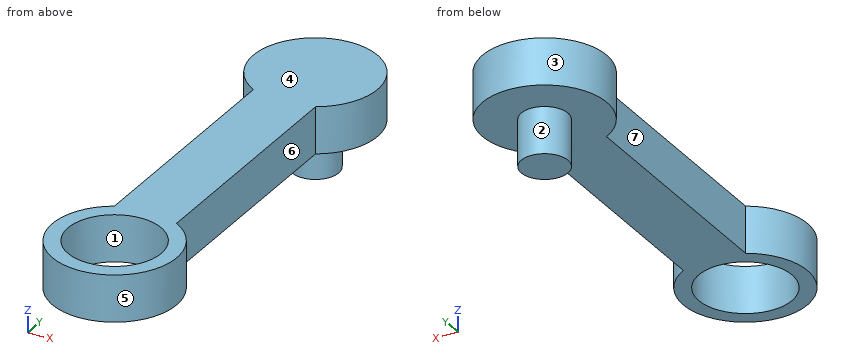
Autodesk Inventor part; units mm, degrees
ref_plane "YZ Plane" through (0, 0, 0) normal (1, 0, 0) x (0, 1, 0)
ref_plane "XZ Plane" through (0, 0, 0) normal (0, 1, 0) x (-1, 0, 0)
ref_plane "XY Plane" through (0, 0, 0) normal (0, 0, 1) x (1, 0, 0)
sketch "Sketch1" plane through (0, 0, 0) normal (0, 0, 1) x (1, 0, 0)
  arc A0 (-4, -15.5718) -> (4, -15.5718) centre (0, -22.5) ccw
  arc A1 (4, 15.5718) -> (-4, 15.5718) centre (0, 22.5) ccw
  line L0 (-4, 15.5718) -> (-4, -15.5718)
  line L1 (4, 15.5718) -> (4, -15.5718)
  circle A2 centre (0, 22.5) radius 3
  circle A3 centre (0, -22.5) radius 6
  point P0 (0, 0)
  dimension "d0" = 45
  dimension "d1" = 22.5
  dimension "d2" = 8
  dimension "d3" = 4
  dimension "d6" = 8
  dimension "d7" = 8
  dimension "d8" = 12
  dimension "d9" = 6
extrude "Extrusion1" add sketch "Sketch1" against normal blind 6
extrude "Extrusion2" add sketch "Sketch1" against normal blind 12 contours A2
properties part number "204"
Geometry: final body of the model. Coordinates: model frame, mm. Face numbers are marked on the shaded views. A direction names the side the tool comes from. Round coordinates to 2 decimals unless told otherwise and drop trailing zeros. Write each loop counter-clockwise with the first axis right and the second up, starting at its lowest first coordinate (ties: lowest second). Pieces come first, ordered by that corner, then holes. Notation, with made-up numbers: M 86.5,-3.5 L 131.5,-3.5 A26 ccw 131.5,33.5 Z; hole C 21.25,79.5 d4. An arc over 180 degrees is marked long. Answer in a Markdown table with one row per item. Add a question column.
(1) Cut plane B-B, the plane x = 0. Return the cut outline in (y, z), then the cut area to 3 significant figures.
(2) Cut plane C-C, the plane y = 22.5. Return the cut outline in (x, z).
(3) Draft query along Y for the marked faces 1, 2, 3 and 4. Return one class per face: pulls with the +Y half, pulls with the -Y half, needs draft (parallel to the pull), parting line crosses it, or undercut.
(4) Reachability of the marked faces 5, 6 and 7 from +Z, -Z, +X, -X, +Y, -Y: full face, straight path, thin tool, end or side. Return the list, or none.
(5) Ray query, L1, parallel to Y at x = 0, z = -2.55; L2, parallel to Z at x = -6, y = 18; L3, parallel to Y at x = 3.75, z = -1.25. Return the intervals inside material, ascending.
(6) Cut plane D-D, the plane z = -3. Return the cut outline in (x, y).
(7) Contact query for flat-ended pins moving along their axis: pin 1 (1.8 mm diameter, centred on y = -0.5, z = -1.5, fed in from +X); pin 2 (5 mm diameter, centred on y = 5, z = -3.5, fed in from -X); pin 3 (6 mm diameter, centred on y = -9.5, z = -10, fed in from -X); pin 4 (8 mm diameter, centred on x = -5, y = 6.5, fed in from -Z). Output: stop coordinate, or through.
(8) Cut plane A-A, the plane y = -22.5. Return the cut outline in (x, z), then the cut area to 3 significant figures.
Established:
| question | item | result |
|---|---|---|
| 1 | outline | M -30.5,-6 L -28.5,-6 L -28.5,0 L -30.5,0 Z; M -16.5,-6 L 19.5,-6 L 19.5,-12 L 25.5,-12 L 25.5,-6 L 30.5,-6 L 30.5,0 L -16.5,0 Z |
| 1 | area | 330 mm² |
| 2 | outline | M -8,-6 L -3,-6 L -3,-12 L 3,-12 L 3,-6 L 8,-6 L 8,0 L -8,0 Z |
| 3 | face 1 | undercut |
| 3 | face 2 | parting line crosses it |
| 3 | face 3 | undercut |
| 3 | face 4 | needs draft |
| 4 | face 5 | +Z, -Z |
| 4 | face 6 | +Z, -Z, +X |
| 4 | face 7 | +Z, -Z, -X |
| 5 | L1 | -30.5 to -28.5, -16.5 to 30.5 |
| 5 | L2 | -6 to 0 |
| 5 | L3 | -29.57 to -27.18, -17.82 to 29.57 |
| 6 | outline | M -4,-15.57 A8 ccw long 4,-15.57 L 4,15.57 A8 ccw long -4,15.57 Z; hole C 0,-22.5 d12 |
| 7 | pin 1 | x = 4 |
| 7 | pin 2 | x = -4 |
| 7 | pin 3 | through |
| 7 | pin 4 | z = -6 |
| 8 | outline | M -8,-6 L -6,-6 L -6,0 L -8,0 Z; M 6,-6 L 8,-6 L 8,0 L 6,0 Z |
| 8 | area | 24.0 mm² |
